from build123d import *

# Parameters (mm, degrees)
SKETCH1_W           = 50
SKETCH1_H           = 80
SKETCH1_R           = 3
BOSS_EXTRUDE1_DEPTH = 9.5
SKETCH2_W           = 80.10102192
SKETCH2_H           = 35
CUT_EXTRUDE1_DEPTH  = 6
SKETCH3_R           = 3
CUT_EXTRUDE2_DEPTH  = 48.549973712
CHAMFER1_SIZE       = 1


with BuildPart() as part:
    # Sketch1 → Boss-Extrude1 (new body)
    with BuildSketch(Plane(origin=(0, 0, 0), x_dir=(1, 0, 0), z_dir=(0, 1, 0))):
        Rectangle(SKETCH1_W, SKETCH1_H)
        with Locations(Location((-15, 30, 0), (0, 0, 270))):
            Circle(SKETCH1_R, mode=Mode.SUBTRACT)
        with Locations(Location((15, 30, 0), (0, 0, 90))):
            Circle(SKETCH1_R, mode=Mode.SUBTRACT)
        with Locations(Location((-15, -30, 0), (0, 0, 90))):
            Circle(SKETCH1_R, mode=Mode.SUBTRACT)
        with Locations(Location((15, -30, 0), (0, 0, 270))):
            Circle(SKETCH1_R, mode=Mode.SUBTRACT)
    extrude(amount=BOSS_EXTRUDE1_DEPTH)

    # Sketch2 → Cut-Extrude1 (cut)
    with BuildSketch(Plane.XZ):
        Rectangle(SKETCH2_W, SKETCH2_H)
    extrude(amount=-CUT_EXTRUDE1_DEPTH, mode=Mode.SUBTRACT)

    # Sketch3 → Cut-Extrude2 (cut, through all)
    with BuildSketch(Plane.XZ.offset(-6)):
        with Locations(Location((-9, 0, 0), (0, 0, 270))):
            Circle(SKETCH3_R)
        with Locations(Location((9, 0, 0), (0, 0, 270))):
            Circle(SKETCH3_R)
    extrude(amount=-CUT_EXTRUDE2_DEPTH, mode=Mode.SUBTRACT)

    # Chamfer1
    chamfer1_edges = [part.edges().sort_by_distance(p)[0] for p in [
        (0, 6, -17.5),
        (0, 6, 17.5),
    ]]
    chamfer(chamfer1_edges, length=CHAMFER1_SIZE)


solid = part.part
Can you work these out from the model? Positions are in its coordinate system, mm. A direction names the side the tool comes from. Coordinates: 2 decimals unless noted, no trailing zeros. Order: outer loops, then holes, each group sorted by start corner. A loop starts at its lowest first (then second) coordinate and runs counter-clockwise, first axis right, second up. Notation, with made-up numbers: M 58.5,-17.5 L 97.5,-17.5 A12 cw 97.5,3.5 Z; hole C 25,56 d8. An arc over 180 degrees is marked long. Write item = value, one per line.
(1) Suppose I cut it at D-D on x = 15. Please give me the cut outline in (y, z).
Results are:
outline = M 0,-40 L 9.5,-40 L 9.5,-33 L 0,-33 Z; M 0,-27 L 9.5,-27 L 9.5,27 L 0,27 L 0,17.5 L 5,17.5 L 6,16.5 L 6,-16.5 L 5,-17.5 L 0,-17.5 Z; M 0,33 L 9.5,33 L 9.5,40 L 0,40 Z
(2) Suppose I cut it at C-C on x = 9. Please give me the cut outline in (y, z), plus the area to 3 significant figures.
Results are:
outline = M 0,-40 L 9.5,-40 L 9.5,-3 L 6,-3 L 6,-16.5 L 5,-17.5 L 0,-17.5 Z; M 0,17.5 L 5,17.5 L 6,16.5 L 6,3 L 9.5,3 L 9.5,40 L 0,40 Z
area = 530 mm2
(3) Suppose I cut it at B-B on z = -30. Please give me the cut outline in (x, y).
Results are:
outline = M -25,0 L -18,0 L -18,9.5 L -25,9.5 Z; M -12,0 L 12,0 L 12,9.5 L -12,9.5 Z; M 18,0 L 25,0 L 25,9.5 L 18,9.5 Z
(4) I need wall thicknesses on line 1 along X through (y, z) = (3, 30); line 2 along X through (y, z) = (8.75, 0); line 3 along Z through (x, y) = (19.5, 4.75). Which ranges of each line are inside material? Lowest first, please. Write a range as [from, to].
Results are:
line_1 = [-25, -18], [-12, 12], [18, 25]
line_2 = [-25, -12], [-6, 6], [12, 25]
line_3 = [-40, -17.5], [17.5, 40]
(5) If we mould it in two halves opening along Z, with no side actions, what happens to faces 1 (the face through (0, 5, 40)), 2 (the face through (0, 6, 0)), 3 (the face through (0, 0, 29))? For each: pulls with the +Z half, pulls with the -Z half, needs draft (parallel to the pull), parting line crosses it, or undercut.
Results are:
face_1 = pulls with the +Z half
face_2 = undercut
face_3 = needs draft
(6) Suppose I cut it at A-A on y = 2. Please give me the cut outline in (x, z).
Results are:
outline = M -25,-40 L 25,-40 L 25,-17.5 L -25,-17.5 Z; M -25,17.5 L 25,17.5 L 25,40 L -25,40 Z; hole C -15,-30 d6; hole C -15,30 d6; hole C 15,-30 d6; hole C 15,30 d6
(7) For faces 4 (the face through (-13.2, 4.7, 32.4)), 5 (the face through (0, 2, -17.5)), which set-ups out of +Z, -Z, +X, -X, +Y, -Y let a thin tool reach every point of the face, with its end or its side?
Results are:
face_4 = +Y, -Y
face_5 = +X, -X, -Y
(8) For pin 1 Ø16.5 at (x, z) = (-3.5, -7.5) entering from -Y, with a flat end and sliding along its axis, tell me the tip position at first contact or that it passes through.
Results are:
pin_1 = 6
